Read the model definition and answer for the solid it produces. Units are mm, in the model's axes. A direction names the side the tool comes from. Coordinates: 2 decimals unless noted, no trailing zeros. Write each loop counter-clockwise with the first axis right and the second up, starting at its lowest first coordinate (ties: lowest second). Pieces come first, ordered by that corner, then holes.
1) Find the intervals of material crossed by line 1 (X direction, y = 12.75, z = 0.2); line 2 (X direction, y = -9, z = 3.1); line 3 (Y direction, x = 18.5, z = 2.8), in increasing order.
2) The part is cut by section B-B (x = 19.5). Determine the outline of the cut face in (y, z).
3) Each of these flat-tipped pins is pushed along its axis until it touches: pin 1 Ø0.5 at (y, z) = (-3, 2.5) entering from +X; pin 2 Ø1.4 at (y, z) = (-4.5, 2.5) entering from +X; pin 3 Ø0.9 at (y, z) = (-1, 3.5) entering from -X; pin 4 Ø0.5 at (x, z) = (1.5, 3) entering from -Y. Where does it stop, or does it pass through?
4) Determine the mould class of faces 5 (the face through (0, 11.6, 3)), 6 (the face through (23.6, 0, 3)), 7 (the face through (-25, 0, 1)) for opening direction X: +X half, -X half, draft (parallel to the pull), parting line (faces both ways), or undercut.
5) The part is cut by section A-A (y = -8.5). Determine the outline of the cut face in (x, z).
6) Which of the six approach directions +Z, -Z, +X, -X, +Y, -Y give full straight-line access (tool end or side, diameter ignored) to faces 1 (the face through (-10.521, 12.517, 1.011)), 2 (the face through (0, 0, 2)), 3 (the face through (0, 12.6, 3)), 4 (the face through (-12, -13, 1))?
7) The part is cut by section C-C (y = -5.25). Determine the outline of the cut face in (x, z), then the cut area to 3 significant figures.
from build123d import *

# Parameters (mm, degrees)
F0_W      = 50
F0_H      = 27
F1_DEPTH  = 2
F2_W      = 1
F2_H      = 23.2
F2_H_2    = 0.3
F3_DEPTH  = 1.8
F4_R      = 1.25
F5_DEPTH  = 2
F11_DEPTH = 3
F12_DEPTH = 3


with BuildPart() as f1:
    # F0 (on Top) → F1 (new body)
    with BuildSketch(Plane.XY):
        Rectangle(F0_W, F0_H)
    extrude(amount=F1_DEPTH)

    # F2 (on face) → F3 (join)
    with BuildSketch(Plane.XY.offset(2)):
        with Locations((23.1, 0)):
            Rectangle(F2_W, F2_H)
        with Locations((23.1, 11.75)):
            Rectangle(F2_W, F2_H_2)
        Polygon((-22.6, 11.6), (22.6, 11.6), (22.6, 11.9), (23.6, 11.9), (23.6, 12.6), (-23.6, 12.6), (-23.6, 11.9), (-22.6, 11.9), align=None)
        with Locations((23.1, -11.75)):
            Rectangle(F2_W, F2_H_2)
        with Locations((-23.1, 0)):
            Rectangle(F2_W, F2_H)
        with Locations((-23.1, 11.75)):
            Rectangle(F2_W, F2_H_2)
        Polygon((22.6, -11.9), (22.6, -11.6), (-22.6, -11.6), (-22.6, -11.9), (-23.6, -11.9), (-23.6, -12.6), (23.6, -12.6), (23.6, -11.9), align=None)
        with Locations((-23.1, -11.75)):
            Rectangle(F2_W, F2_H_2)
    extrude(amount=F3_DEPTH)

    # F4 (on face) → F5 (cut)
    with BuildSketch(Plane(origin=(0, 0, 0), x_dir=(1, 0, 0), z_dir=(0, 0, -1))):
        with Locations((-14.5, 8.5)):
            Circle(F4_R)
        with Locations((19.5, -5)):
            Circle(F4_R)
    extrude(amount=-F5_DEPTH, mode=Mode.SUBTRACT)

    # F9 (on offset) → F11 (cut)
    with BuildSketch(Plane.YZ.offset(12)):
        Polygon((0, -11.506825), (-13.72761, 2.220785), (-13.72761, -11.823715), (0, -11.823715), (13.72761, -11.823715), (13.72761, 2.220785), align=None)
    extrude(amount=-F11_DEPTH, mode=Mode.SUBTRACT)

    # F10 (on offset) → F12 (cut)
    with BuildSketch(Plane.YZ.offset(-12)):
        Polygon((0, -11.506825), (-13.72761, 2.220785), (-13.72761, -11.823715), (0, -11.823715), (13.72761, -11.823715), (13.72761, 2.220785), align=None)
    extrude(amount=F12_DEPTH, mode=Mode.SUBTRACT)


solid = f1.part
Reported:
1. line 1: x = -25 to -12, -9 to 9, 12 to 25
1. line 2: x = -23.6 to -22.6, 22.6 to 23.6
1. line 3: y = -12.6 to -11.6, 11.6 to 12.6
2. outline: (-13.5, 0) - (3.75, 0) - (3.75, 2) - (-11.6, 2) - (-11.6, 3.8) - (-12.6, 3.8) - (-12.6, 2) - (-13.5, 2) - close; (6.25, 0) - (13.5, 0) - (13.5, 2) - (12.6, 2) - (12.6, 3.8) - (11.6, 3.8) - (11.6, 2) - (6.25, 2) - close
3. pin 1: stops at x = 23.6
3. pin 2: stops at x = 25
3. pin 3: stops at x = -23.6
3. pin 4: stops at y = -12.6
4. face 5: undercut
4. face 6: +X half
4. face 7: -X half
5. outline: (-25, 0) - (-15.75, 0) - (-15.75, 2) - (-22.6, 2) - (-22.6, 3.8) - (-23.6, 3.8) - (-23.6, 2) - (-25, 2) - close; (-13.25, 0) - (25, 0) - (25, 2) - (23.6, 2) - (23.6, 3.8) - (22.6, 3.8) - (22.6, 2) - (-13.25, 2) - close
6. face 1: -Z, +Y
6. face 2: +Z
6. face 3: +Z, +X, -X, +Y
6. face 4: -Z, -Y
7. outline: (-25, 0) - (25, 0) - (25, 2) - (23.6, 2) - (23.6, 3.8) - (22.6, 3.8) - (22.6, 2) - (-22.6, 2) - (-22.6, 3.8) - (-23.6, 3.8) - (-23.6, 2) - (-25, 2) - close
7. area: 104 mm2
